Autodesk Inventor part; units mm, degrees
ref_plane "Work Plane1" through (25.5715, 0, 85.2393) normal (0.7822, 0, 0.6231) x (0, 1, 0)
ref_plane "Work Plane2" through (-25.5715, 3, 0) normal (0, -1, 0) x (1, 0, 0)
ref_plane "YZ Plane" through (0, 0, 0) normal (1, 0, 0) x (0, 1, 0)
sketch "Sketch1" plane through (0, 0, 0) normal (0, 0, 1) x (1, 0, 0)
  circle A0 centre (-16, 13) radius 1.75
  circle A1 centre (16, 13) radius 1.75
  line L0 (-16, 13) -> (16, 13) construction
  line L1 (0, 13) -> (0, 0) construction
  line L2 (0, 0) -> (-25.5715, 0)
  line L3 (-25.5715, 0) -> (-25.5715, 6)
  line L4 (-25.5715, 6) -> (-20.5, 6)
  line L5 (-20.5, 6) -> (-20.5, 13)
  line L6 (-16, 17.5) -> (0, 17.5)
  arc A2 (-16, 17.5) -> (-20.5, 13) centre (-16, 13) ccw
  circle A3 centre (16, 13) radius 1.75
  line L7 (0, 0) -> (25.5715, 0)
  line L8 (25.5715, 0) -> (25.5715, 6)
  line L9 (25.5715, 6) -> (20.5, 6)
  line L10 (20.5, 6) -> (20.5, 13)
  line L11 (16, 17.5) -> (0, 17.5)
  arc A4 (20.5, 13) -> (16, 17.5) centre (16, 13) ccw
  dimension "d0" = 3.5
  dimension "d1" = 3.5
  dimension "d2" = 32
  dimension "d3" = 13
  dimension "d4" = 25.5715
  dimension "d5" = 6
  dimension "d18" = 4.5
extrude "Extrusion1" add sketch "Sketch1" along normal blind 4.5
sketch "Sketch2" plane through (-25.5715, 0, 0) normal (0, -1, 0) x (1, 0, 0)
  line L0 (0, 0) -> (51.143, 0)
  line L1 (51.143, 0) -> (51.143, 4.5)
  line L2 (0, 4.5) -> (51.143, 4.5)
  line L3 (0, 0) -> (0, 4.5)
  line L4 (0, 4.5) -> (0, 44.5)
  line L5 (0, 44.5) -> (51.143, 85.2393)
  line L6 (51.143, 85.2393) -> (51.143, 4.5)
  line L7 (46.143, 4.5) -> (46.143, 74.864)
  line L8 (46.143, 74.864) -> (5, 42.0904)
  line L9 (5, 42.0904) -> (5, 4.5)
  line L10 (5, 4.5) -> (46.143, 23.2952) construction
  line L11 (5, 42.0904) -> (46.143, 23.2952) construction
  line L12 (5, 23.2952) -> (46.143, 23.2952) construction
  line L13 (5, 4.5) -> (0, 4.5)
  line L14 (46.143, 4.5) -> (51.143, 4.5)
  line L15 (7.1928, 43.8372) -> (46.143, 26.0437)
  line L16 (5, 39.3419) -> (40.1265, 23.2952)
  line L17 (40.1265, 23.2952) -> (5, 7.2485)
  line L18 (46.143, 20.5467) -> (11.0165, 4.5)
  line L19 (5, 7.2485) -> (5, 4.5)
  point P0 (25.5715, 0)
  dimension "d9" = 128.54
  dimension "d10" = 40
  dimension "d11" = 5
  dimension "d14" = 2.5
  dimension "d15" = 2.5
extrude "Extrusion2" add sketch "Sketch2" against normal blind 6 contours L4 L5 L6 L2 L7 L8 L9 | L9 L17 L16 L8 L15 L7 L18 L2
ref_plane "Work Plane1" through (25.5715, 0, 85.2393) normal (0.7822, 0, 0.6231) x (0, 1, 0)
sketch "Sketch4" plane through (25.5715, 0, 85.2393) normal (0.7822, 0, 0.6231) x (0, 1, 0)
  line L0 (0, -66.6719) -> (6, -66.6719)
  line L1 (6, -66.6719) -> (6, 0)
  line L2 (0, 0) -> (6, 0)
  line L3 (0, -66.6719) -> (0, 0)
  line L4 (0, -1.1) -> (1.2, -3.3)
  line L5 (1.2, -3.3) -> (0, -3.3)
  line L6 (3, 0) -> (3, -3.4483) construction
  point P0 (0, -50.7393)
  dimension "d29" = 1.1
  dimension "d30" = 3.3
  dimension "d31" = 3.6
extrude "Extrusion4" cut sketch "Sketch4" against normal blind 64 contours L3 L4 L5
ref_plane "Work Plane2" through (-25.5715, 3, 0) normal (0, -1, 0) x (1, 0, 0)
mirror "Mirror1" about plane through (-25.5715, 3, 0) normal (0, -1, 0) of "Extrusion4"
equation "\"d14\" = 0.5 * d11"
equation "\"d15\" = d14"
properties part number "Base_ScreenHolder_L"
Geometry check sheet. Reference: the model listing, model coordinates, mm. A direction names the side the tool comes from. Round coordinates to 2 decimals unless told otherwise and drop trailing zeros. Write each loop counter-clockwise with the first axis right and the second up, starting at its lowest first coordinate (ties: lowest second). Pieces come first, ordered by that corner, then holes. Notation, with made-up numbers: (-5, 50) -> (7, 50) arc R16 cw to (7, 69) -> close; hole circle Ø8 at (-11.5, 22). An arc over 180 degrees is marked (long way). One line per item, written item: value. Start each with the question number.
(1) Cross-section at B-B, the plane z = 57. Record the cut outline in (x, y), and give its area (3 significant figures).
(2) Go/stop test with flat-tipped pins: pin 1 Ø10 at (x, y) = (3, 14) entering from +Z; pin 2 Ø5 at (y, z) = (9, 2) entering from +X; pin 3 Ø1.3 at (y, z) = (8, 3) entering from -X; pin 4 Ø1.5 at (x, y) = (-8, 14.5) entering from -Z. Record where each tip stops, or that it passes through.
(3) Cross-section at D-D, the plane z = 9. Record the cut outline in (x, y).
(4) Cross-section at A-A, the plane x = -19.5. Record the cut outline in (y, z), and give its area (3 significant figures).
(5) Access from +Z, -Z, +X, -X, +Y, -Y to the whole of each face (thin tool, end or side, straight path). Record for faces 1 (the flat face through (20.5, 9, 2)), 2 (the flat face through (3.254, 2.958, 12.636)), 3 (the flat face through (25.572, 3, 42)).
(6) Draft check along Z on faces 4 (the flat face through (0, 9, 0)), 5 (the flat face through (-20.572, 3, 24)), 6 (the flat face through (4, 6, 33)). Enter one of: +Z half, -Z half, draft (parallel to the pull), parting line (faces both ways), or undercut.
(7) Cross-section at C-C, the plane x = -11.5. Record the cut outline in (y, z).
(8) Scan lines: line 1 (Y direction, x = -16, z = 3); line 2 (Y direction, x = 8, z = 29.5); line 3 (Z direction, x = -12, y = 16). Record each from-to range of solid material in increasing order. Write a range as [from, to].
Answer:
1. outline: (-9.88, 0) -> (-8.11, 0) -> (-4.58, 1.2) -> (-4.58, 0) -> (-1.85, 0) -> (-1.85, 6) -> (-4.58, 6) -> (-4.58, 4.8) -> (-8.11, 6) -> (-9.88, 6) -> close; (20.57, 0) -> (25.57, 0) -> (25.57, 6) -> (20.57, 6) -> close
1. area: 73.9 mm²
2. pin 1: z = 4.5
2. pin 2: x = 20.5
2. pin 3: x = -20.5
2. pin 4: z = 0
3. outline: (-25.57, 0) -> (-20.57, 0) -> (-20.57, 6) -> (-25.57, 6) -> close; (-16.74, 0) -> (-4.7, 0) -> (-4.7, 6) -> (-16.74, 6) -> close; (20.57, 0) -> (25.57, 0) -> (25.57, 6) -> (20.57, 6) -> close
4. outline: (0, 0) -> (15.83, 0) -> (15.83, 4.5) -> (6, 4.5) -> (6, 7.74) -> (0, 7.74) -> close; (0, 38.85) -> (6, 38.85) -> (6, 45.12) -> (4.8, 45.12) -> (6, 47.93) -> (6, 49.34) -> (0, 49.34) -> (0, 47.93) -> (1.2, 45.12) -> (0, 45.12) -> close
4. area: 150 mm²
5. face 1: +Z, -Z, +X, +Y
5. face 2: +Y, -Y
5. face 3: +Z, -Z, +X, +Y, -Y
6. face 4: -Z half
6. face 5: undercut
6. face 6: draft
7. outline: (0, 0) -> (17.5, 0) -> (17.5, 4.5) -> (0, 4.5) -> close; (0, 5.9) -> (6, 5.9) -> (6, 11.39) -> (0, 11.39) -> close; (0, 35.2) -> (6, 35.2) -> (6, 40.69) -> (0, 40.69) -> close; (0, 49.32) -> (6, 49.32) -> (6, 51.49) -> (4.8, 51.49) -> (6, 54.3) -> (6, 55.71) -> (0, 55.71) -> (0, 54.3) -> (1.2, 51.49) -> (0, 51.49) -> close
8. line 1: [0, 11.25], [14.75, 17.5]
8. line 2: [0, 6]
8. line 3: [0, 4.5]
